Verification items for the finished model (mm, model axes). A direction names the side the tool comes from. Give positions to 0.01 mm unless a question says otherwise; leave off trailing zeros. Order: outer loops, then holes, each group sorted by start corner. A loop starts at its lowest first (then second) coordinate and runs counter-clockwise, first axis right, second up.
Autodesk Inventor part; units mm, degrees
ref_plane "YZ Plane" through (0, 0, 0) normal (1, 0, 0) x (0, 1, 0)
ref_plane "XZ Plane" through (0, 0, 0) normal (0, 1, 0) x (-1, 0, 0)
ref_plane "XY Plane" through (0, 0, 0) normal (0, 0, 1) x (1, 0, 0)
sketch "스케치1" plane through (0, 0, 0) normal (0, 1, 0) x (-1, 0, 0)
  line L0 (75, 10) -> (-75, 10)
  line L1 (-75, 10) -> (-75, -10)
  line L2 (-75, -10) -> (75, -10)
  line L3 (75, -10) -> (75, 10)
  line L4 (75, 10) -> (-75, -10) construction
  line L5 (-75, 10) -> (75, -10) construction
  circle A0 centre (35, 0) radius 2.25
  line L6 (105, 0) -> (-105, 0)
  circle A1 centre (-35, 0) radius 2.25
  point P0 (0, 0)
  point P1 (-75, 0)
  dimension "d0" = 150
  dimension "d1" = 20
  dimension "d4" = 4.5
  dimension "d5" = 40
  dimension "d6" = 4.5
  dimension "d7" = 40
extrude "돌출1" add sketch "스케치1" along normal blind 3
sketch "스케치4" plane through (0, 0, 0) normal (0, -1, 0) x (1, 0, 0)
  line L0 (-35, -2) -> (-35, 2) construction
  line L1 (-33, -2) -> (-33, 2)
  line L2 (-37, 2) -> (-37, -2)
  arc A0 (-37, -2) -> (-33, -2) centre (-35, -2) ccw
  arc A1 (-33, 2) -> (-37, 2) centre (-35, 2) ccw
  line L3 (35, -2) -> (35, 2) construction
  line L4 (37, -2) -> (37, 2)
  line L5 (33, 2) -> (33, -2)
  arc A2 (33, -2) -> (37, -2) centre (35, -2) ccw
  arc A3 (37, 2) -> (33, 2) centre (35, 2) ccw
  line L6 (-75, 10) -> (75, 10)
  line L7 (75, 10) -> (75, -10)
  line L8 (-75, -10) -> (-75, 10)
  line L9 (75, -10) -> (-75, -10)
  line L10 (68, 2) -> (68, -2) construction
  line L11 (66, 2) -> (66, -2)
  line L12 (70, -2) -> (70, 2)
  arc A4 (70, 2) -> (66, 2) centre (68, 2) ccw
  arc A5 (66, -2) -> (70, -2) centre (68, -2) ccw
  line L13 (-65, -2) -> (-65, 2) construction
  line L14 (-63, -2) -> (-63, 2)
  line L15 (-67, 2) -> (-67, -2)
  arc A6 (-67, -2) -> (-63, -2) centre (-65, -2) ccw
  arc A7 (-63, 2) -> (-67, 2) centre (-65, 2) ccw
  point P0 (-35, 0)
  point P1 (35, 0)
  point P2 (68, 0)
  point P3 (-65, 0)
  point P4 (75, 0)
  point P5 (75, 0)
  point P6 (-75, 0)
  point P7 (-75, 0)
  dimension "d14" = 4
  dimension "d15" = 4
  dimension "d16" = 4
  dimension "d17" = 4
  dimension "d18" = 10
  dimension "d19" = 40
  dimension "d20" = 10
  dimension "d21" = 40
  dimension "d28" = 4
  dimension "d29" = 4
  dimension "d30" = 4
  dimension "d31" = 4
  dimension "d32" = 0
  dimension "d33" = 7
  dimension "d34" = 0
  dimension "d35" = 10
extrude "돌출3" cut sketch "스케치4" against normal blind 10 contours A0 L2 A1 L1 | A2 L5 A3 L4 | A4 L12 A5 L11 | A6 L15 A7 L14
properties part number "발받침대위,아래"
(1) Release check for a two-part mould opening along Z. For faces 3 (the flat face through (1, 1, -10)), 4 (the cylindrical face through (-35, 1, -4)), 5 (the flat face through (1, 0, 0)) record: pulls with the +Z half, pulls with the -Z half, needs draft (parallel to the pull), parting line crosses it, or undercut.
Solved:
face 3: pulls with the -Z half
face 4: undercut
face 5: needs draft
(2) Set-up check for faces 1 (the cylindrical face through (68, 1, 4)), 2 (the flat face through (1, 3, 0)): record each of +Z, -Z, +X, -X, +Y, -Y from which the full face is reachable in a straight line by a thin tool's end or side.
Solved:
face 1: +Y, -Y
face 2: +Z, -Z, +X, -X, +Y
(3) Section check B-B, the plane z = 0. Enter the section's corners in (x, y), then the cut area to 3 significant figures.
Solved:
outline: (-75, 0) - (-67, 0) - (-67, 3) - (-75, 3) - close; (-63, 0) - (-37, 0) - (-37, 3) - (-63, 3) - close; (-33, 0) - (33, 0) - (33, 3) - (-33, 3) - close; (37, 0) - (66, 0) - (66, 3) - (37, 3) - close; (70, 0) - (75, 0) - (75, 3) - (70, 3) - close
area: 402 mm2
(4) Section check C-C, the plane y = 1.05. Enter the section's corners in (x, z).
Solved:
outline: (-75, -10) - (75, -10) - (75, 10) - (-75, 10) - close; hole (-67, -2) arc R2 ccw to (-63, -2) - (-63, 2) arc R2 ccw to (-67, 2) - close; hole (-37, -2) arc R2 ccw to (-33, -2) - (-33, 2) arc R2 ccw to (-37, 2) - close; hole (33, -2) arc R2 ccw to (37, -2) - (37, 2) arc R2 ccw to (33, 2) - close; hole (66, -2) arc R2 ccw to (70, -2) - (70, 2) arc R2 ccw to (66, 2) - close
(5) Scan lines: line 1 (X direction, y = 2.15, z = -2.25); line 2 (X direction, y = 1, z = 2.75); line 3 (Z direction, x = -66, y = 1.55). Record each from-to range of solid material in increasing order.
Solved:
line 1: x = -75 to -66.98, -63.02 to -36.98, -33.02 to 33.02, 36.98 to 66.02, 69.98 to 75
line 2: x = -75 to -66.85, -63.15 to -36.85, -33.15 to 33.15, 36.85 to 66.15, 69.85 to 75
line 3: z = -10 to -3.73, 3.73 to 10
(6) Section check A-A, the plane x = -65. Enter the section's corners in (y, z), then the cut area to 3 significant figures.
Solved:
outline: (0, -10) - (3, -10) - (3, -4) - (0, -4) - close; (0, 4) - (3, 4) - (3, 10) - (0, 10) - close
area: 36.0 mm2
